Part model, mm, in its own coordinate system. Face numbers are marked on the shaded views. A direction names the side the tool comes from. Round coordinates to 2 decimals unless told otherwise and drop trailing zeros. Loops run counter-clockwise (first coordinate to the right, second up) from the corner with the lowest first, then second, coordinate; pieces in that order, holes last.
from build123d import *

# Parameters (mm, degrees)
SKETCH008_W     = 90.71
SKETCH008_H     = 53.7
SKETCH008_R     = 1.475
SKETCH008_W_2   = 76.71
SKETCH008_H_2   = 51
PAD002_DEPTH    = 17.5
FILLET001_R     = 3
SKETCH009_R     = 0.8
POCKET005_DEPTH = 5
SKETCH010_W     = 40
SKETCH010_H     = 13.5
POCKET006_DEPTH = 7
SKETCH012_W     = 6
SKETCH012_H     = 51
PAD003_DEPTH    = 1
CHAMFER_SIZE    = 5.99
SKETCH015_R     = 1.25
PAD004_DEPTH    = 2
FILLET005_R     = 1
FILLET006_R     = 1
FILLET007_R     = 2
SKETCH016_W     = 1.25
SKETCH016_H     = 4.821428
POCKET009_DEPTH = 1.5
CHAMFER002_SIZE = 0.5


with BuildPart() as part:
    # Sketch008 (on Face1 of CopyCopyHole) → Pad002 (new body)
    with BuildSketch(Plane(origin=(0, 0, -11.25), x_dir=(1, 0, 0), z_dir=(0, 0, -1))):
        with Locations((-2.23, 0)):
            Rectangle(SKETCH008_W, SKETCH008_H)
        with Locations((-43.585, 22.85)):
            Circle(SKETCH008_R, mode=Mode.SUBTRACT)
        with Locations((-43.585, -22.85)):
            Circle(SKETCH008_R, mode=Mode.SUBTRACT)
        with Locations((39.125, 22.85)):
            Circle(SKETCH008_R, mode=Mode.SUBTRACT)
        with Locations((39.125, -22.85)):
            Circle(SKETCH008_R, mode=Mode.SUBTRACT)
        with Locations((-2.23, 0)):
            Rectangle(SKETCH008_W_2, SKETCH008_H_2, mode=Mode.SUBTRACT)
    extrude(amount=PAD002_DEPTH)

    # Fillet001
    fillet001_edges = [part.edges().sort_by_distance(p)[0] for p in [
        (43.125, 26.85, -20),
        (-47.585, 26.85, -20),
        (-47.585, -26.85, -20),
        (43.125, -26.85, -20),
    ]]
    fillet(fillet001_edges, radius=FILLET001_R)

    # Sketch009 (on Face10 of Fillet001) → Pocket005 (cut)
    with BuildSketch(Plane(origin=(0, 26.85, 0), x_dir=(-1, 0, 0), z_dir=(0, 1, 0))):
        with Locations((-35.175, -17.75)):
            Circle(SKETCH009_R)
        with BuildLine():
            ThreePointArc((-31.775, -18.75), (-29.275, -21.25), (-26.775, -18.75))
            Line((-26.775, -18.75), (-26.775, -11.25))
            ThreePointArc((-26.775, -11.25), (-29.275, -8.75), (-31.775, -11.25))
            Line((-31.775, -18.75), (-31.775, -11.25))
        make_face()
    extrude(amount=-POCKET005_DEPTH, mode=Mode.SUBTRACT)

    # Sketch010 (on Face7 of Fillet001) → Pocket006 (cut)
    with BuildSketch(Plane.YZ.offset(43.125)):
        with Locations((0, -18)):
            Rectangle(SKETCH010_W, SKETCH010_H)
    extrude(amount=-POCKET006_DEPTH, mode=Mode.SUBTRACT)

    # Sketch012 (on Face2 of Pocket006) → Pad003 (join)
    with BuildSketch(Plane.XY.offset(-11.25)):
        with Locations((-37.585, 0)):
            Rectangle(SKETCH012_W, SKETCH012_H)
    extrude(amount=-PAD003_DEPTH)

    # Chamfer
    chamfer_edges = [part.edges().sort_by_distance(p)[0] for p in [
        (-40.585, 0, -12.25),
    ]]
    chamfer(chamfer_edges, length=CHAMFER_SIZE)

    # Sketch015 (on Face9 of Chamfer) → Pad004 (join)
    with BuildSketch(Plane.XY.offset(-11.25)):
        with Locations((-42.585, 16)):
            Circle(SKETCH015_R)
        with Locations((-42.585, -16)):
            Circle(SKETCH015_R)
    extrude(amount=PAD004_DEPTH)

    # Fillet005
    fillet005_edges = [part.edges().sort_by_distance(p)[0] for p in [
        (-43.835, -16, -9.25),
        (-43.835, 16, -9.25),
    ]]
    fillet(fillet005_edges, radius=FILLET005_R)

    # Fillet006
    fillet006_edges = [part.edges().sort_by_distance(p)[0] for p in [
        (36.125, -25.5, -20),
        (-40.585, -25.5, -23.495),
        (-40.585, 25.5, -23.495),
    ]]
    fillet(fillet006_edges, radius=FILLET006_R)

    # Fillet007
    fillet007_edges = [part.edges().sort_by_distance(p)[0] for p in [
        (39.625, 20, -24.75),
        (39.625, -20, -24.75),
    ]]
    fillet(fillet007_edges, radius=FILLET007_R)

    # Sketch016 (on Face9 of Fillet007) → Pocket009 (cut)
    with BuildSketch(Plane.XZ.offset(-20)):
        with Locations((41.5, -18)):
            Rectangle(SKETCH016_W, SKETCH016_H)
    pocket009 = extrude(amount=-POCKET009_DEPTH, mode=Mode.SUBTRACT)

    # Mirrored001: Pocket009 across XZ
    add(pocket009.mirror(Plane.XZ), mode=Mode.SUBTRACT)

    # Chamfer002
    chamfer002_edges = [part.edges().sort_by_distance(p)[0] for p in [
        (29.275, 26.85, -21.25),
    ]]
    chamfer(chamfer002_edges, length=CHAMFER002_SIZE)


solid = part.part
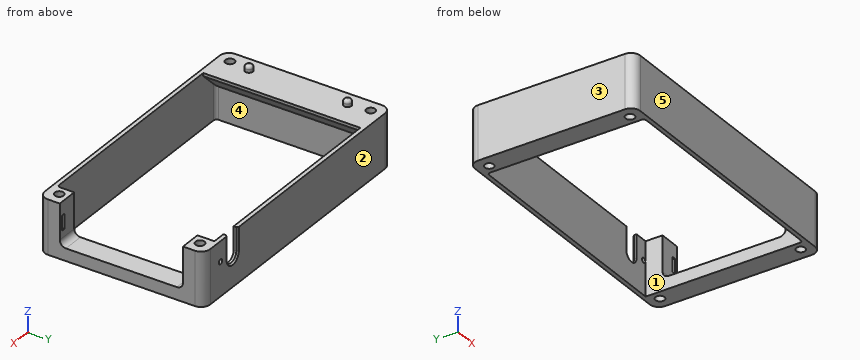
1) Tool access for the marked faces 1 and 2: list every direction of +Z, -Z, +X, -X, +Y, -Y with a clear straight run to the whole face (end or side of a thin tool).
Values:
face 1: +Z, -Z
face 2: +Z, -Z, +X, -X, +Y
2) Wall check: line 1 along X through (y, z) = (22.85, -21.5) (3 decimals); line 2 along Y through (x, z) = (-24.5, -18); line 3 along X through (y, z) = (-21, -19.25) (3 decimals). Give the ranges that are in metal, low to high.
Values:
line 1: x = -47.585 to -45.06, -42.11 to -40.585, 36.125 to 37.65, 40.6 to 43.125
line 2: y = -26.85 to -25.5, 25.5 to 26.85
line 3: x = -47.585 to -40.585, 36.125 to 40.875, 42.125 to 43.125
3) Slice it at B-B, the plane x = 23. Give the cut face in (y, z), then the cut area to 4 significant figures.
Values:
outline: (-26.85, -28.75) - (-25.5, -28.75) - (-25.5, -11.25) - (-26.85, -11.25) - close; (25.5, -28.75) - (26.85, -28.75) - (26.85, -11.25) - (25.5, -11.25) - close
area: 47.25 mm2
4) Drop flat-ended pins along their axis: pin 1 Ø3.5 at (x, y) = (39.5, 25) entering from +Z; pin 2 Ø3.5 at (x, z) = (40.5, -16.5) entering from +Y; pin 3 Ø0.8 at (y, z) = (5.5, -11.5) entering from +X (3 decimals). Give the stop position or say it passes through.
Values:
pin 1: stops at z = -11.25
pin 2: stops at y = 26.85
pin 3: stops at x = -34.585
5) Slice it at A-A, the plane y = 22.85. Give the cut face in (x, z) (3 decimals).
Values:
outline: (-47.585, -28.75) - (-45.06, -28.75) - (-45.06, -11.25) - (-47.585, -11.25) - close; (-42.11, -28.75) - (-40.585, -28.75) - (-40.585, -18.24) - (-34.595, -12.25) - (-34.585, -12.25) - (-34.585, -11.25) - (-42.11, -11.25) - close; (36.125, -28.75) - (37.65, -28.75) - (37.65, -11.25) - (36.125, -11.25) - close; (40.6, -28.75) - (43.125, -28.75) - (43.125, -11.25) - (40.6, -11.25) - close
6) Slice it at C-C, the plane x = -37.5. Give the cut face in (y, z) (3 decimals), then the cut area to 3 significant figures.
Values:
outline: (-26.85, -28.75) - (-25.5, -28.75) - (-25.5, -15.155) - (25.5, -15.155) - (25.5, -28.75) - (26.85, -28.75) - (26.85, -11.25) - (-26.85, -11.25) - close
area: 246 mm2
7) Mould opens along X. For the marked faces 3, 4 and 5 say: released by +X, released by -X, zero draft, split by the parting line, or undercut.
Values:
face 3: released by -X
face 4: undercut
face 5: zero draft
